Can you work these out from the drawing? Everything is in mm from the part's minimum corner. A direction names the side the tool comes from. Round coordinates to 2 decimals unless told otherwise and drop trailing zeros. Write each loop counter-clockwise with the first axis right and the second up, starting at its lowest first coordinate (ties: lowest second). Pieces come first, ordered by that corner, then holes. Notation, with made-up numbers: (1.25, 26.25) - (53.25, 26.25) arc R26 ccw to (53.25, 62.25) - close; hole circle Ø9 at (-36, 2.25). An arc over 180 degrees is marked (long way). One line per item, written item: value. Start each with the question number.
(1) On a 3-axis mill with a long thin cutter (end or side, diameter ignored), from which of +Z, -Z, +X, -X, +Y, -Y can I reach the whole of each face in a straight line? I mean the marked faces 1 and 2. Say none if no direction works.
(2) I want a section at C-C on z = 53.5. List the corners of the cut face in (x, y) for me.
(3) If I drill on L1, parallel to Y at x = 10.75, z = 61.5; L2, parallel to Y at x = 7.5, z = 83; L3, parallel to X at y = 2.5, z = 86, over which ranges is the centre line in solid material (lowest first)? Write a range as from..to.
(4) I want a section at D-D on z = 22. List the corners of the cut face in (x, y) for me.
(5) I want a section at A-A on x = 8. List the corners of the cut face in (y, z) for me.
(6) I'm going to push flat-ended pins straight in: pin 1 Ø6 at (y, z) = (13, 60.5) entering from -X; pin 2 Ø1.5 at (y, z) = (3, 86.5) entering from -X; pin 3 Ø4 at (x, z) = (10, 33.5) entering from -Y. Where does each tip first touch, or does it pass through?
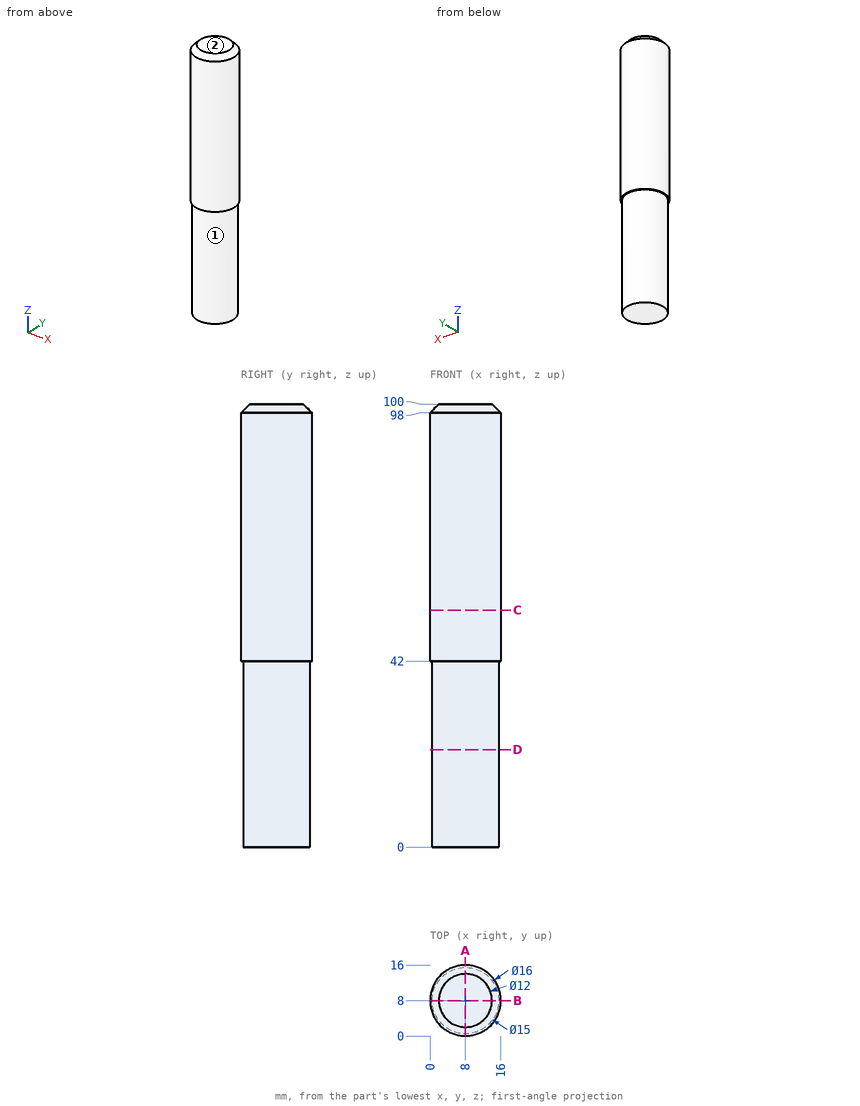
Established:
1. face 1: -Z
1. face 2: +Z, +X, -X, +Y, -Y
2. outline: circle Ø16 at (8, 8)
3. L1: 0.49..15.51
3. L2: 0.02..15.98
3. L3: 2.19..13.81
4. outline: circle Ø15 at (8, 8)
5. outline: (0, 42) - (0.5, 42) - (0.5, 0) - (15.5, 0) - (15.5, 42) - (16, 42) - (16, 98) - (14, 100) - (2, 100) - (0, 98) - close
6. pin 1: x = 0.25
6. pin 2: x = 1.22
6. pin 3: y = 0.5
